```python
from build123d import *

# Parameters (mm, degrees)
F0_W     = 66.675
F0_H     = 125.4125
F0_W_2   = 63.5
F0_H_2   = 63.5
F1_DEPTH = 1.1811
F2_R     = 2.54
F2_R_2   = 6.35
F3_DEPTH = 1.1811
F4_R     = 5.08


with BuildPart() as f1:
    # F0 (on Top) → F1 (new body)
    with BuildSketch(Plane.XY):
        with Locations((0, 62.70625)):
            Rectangle(F0_W, F0_H)
        with Locations((-65.0875, 62.70625)):
            Rectangle(F0_W_2, F0_H)
        with Locations((65.0875, 62.70625)):
            Rectangle(F0_W_2, F0_H)
        with Locations((0, 157.1625)):
            Rectangle(F0_W, F0_H_2)
    extrude(amount=F1_DEPTH)

    # F2 (on face) → F3 (cut, through all)
    with BuildSketch(Plane.XY.offset(1.1811)):
        with BuildLine():
            ThreePointArc((-31.75, 109.5375), (-33.3375, 111.125), (-34.925, 109.5375))
            Line((-34.925, 109.5375), (-34.925, 90.4875))
            ThreePointArc((-34.925, 90.4875), (-33.3375, 88.9), (-31.75, 90.4875))
            Line((-31.75, 90.4875), (-31.75, 109.5375))
        make_face()
        with BuildLine():
            ThreePointArc((-31.75, 72.1995), (-33.3375, 73.787), (-34.925, 72.1995))
            Line((-34.925, 72.1995), (-34.925, 53.1495))
            ThreePointArc((-34.925, 53.1495), (-33.3375, 51.562), (-31.75, 53.1495))
            Line((-31.75, 53.1495), (-31.75, 72.1995))
        make_face()
        with BuildLine():
            ThreePointArc((-31.75, 34.8615), (-33.3375, 36.449), (-34.925, 34.8615))
            Line((-34.925, 34.8615), (-34.925, 15.8115))
            ThreePointArc((-34.925, 15.8115), (-33.3375, 14.224), (-31.75, 15.8115))
            Line((-31.75, 15.8115), (-31.75, 34.8615))
        make_face()
        with BuildLine():
            ThreePointArc((34.925, 34.8615), (33.3375, 36.449), (31.75, 34.8615))
            Line((31.75, 34.8615), (31.75, 15.8115))
            ThreePointArc((31.75, 15.8115), (33.3375, 14.224), (34.925, 15.8115))
            Line((34.925, 15.8115), (34.925, 34.8615))
        make_face()
        with BuildLine():
            ThreePointArc((34.925, 72.1995), (33.3375, 73.787), (31.75, 72.1995))
            Line((31.75, 72.1995), (31.75, 53.1495))
            ThreePointArc((31.75, 53.1495), (33.3375, 51.562), (34.925, 53.1495))
            Line((34.925, 53.1495), (34.925, 72.1995))
        make_face()
        with BuildLine():
            ThreePointArc((34.925, 109.5375), (33.3375, 111.125), (31.75, 109.5375))
            Line((31.75, 109.5375), (31.75, 90.4875))
            ThreePointArc((31.75, 90.4875), (33.3375, 88.9), (34.925, 90.4875))
            Line((34.925, 90.4875), (34.925, 109.5375))
        make_face()
        with BuildLine():
            ThreePointArc((-17.4625, 127), (-19.05, 125.4125), (-17.4625, 123.825))
            Line((-17.4625, 123.825), (-7.9375, 123.825))
            ThreePointArc((-7.9375, 123.825), (-6.35, 125.4125), (-7.9375, 127))
            Line((-7.9375, 127), (-17.4625, 127))
        make_face()
        with BuildLine():
            ThreePointArc((7.9375, 127), (6.35, 125.4125), (7.9375, 123.825))
            Line((7.9375, 123.825), (17.4625, 123.825))
            ThreePointArc((17.4625, 123.825), (19.05, 125.4125), (17.4625, 127))
            Line((17.4625, 127), (7.9375, 127))
        make_face()
        with Locations((-33.3375, 125.4125)):
            Circle(F2_R)
        with Locations((33.3375, 125.4125)):
            Circle(F2_R)
        with Locations((0, 74.6125)):
            Circle(F2_R_2)
    extrude(amount=-F3_DEPTH, mode=Mode.SUBTRACT)

    # F4
    f4_edges = [f1.edges().sort_by_distance(p)[0] for p in [
        (-96.8375, 0, 0.59055),
        (96.8375, 0, 0.59055),
    ]]
    fillet(f4_edges, radius=F4_R)


solid = f1.part
```
Read the model definition and answer for the solid it produces. Units are mm, in the model's axes. Coordinates: 2 decimals unless noted, no trailing zeros. Loops run counter-clockwise (first coordinate to the right, second up) from the corner with the lowest first, then second, coordinate; pieces in that order, holes last. Notation, with made-up numbers: (26.25, 81.5) -> (53.25, 81.5) arc R28 cw to (53.25, 109.5) -> close; hole circle Ø3 at (82.25, 40). An arc over 180 degrees is marked (long way). Return JSON: item names as keys, results as strings.
Item 1: Find section B-B (y = 77). Determine the outline of the cut face in (x, z).
Answers:
{"outline": "(-96.84, 0) -> (-5.88, 0) -> (-5.88, 1.18) -> (-96.84, 1.18) -> close; (5.88, 0) -> (96.84, 0) -> (96.84, 1.18) -> (5.88, 1.18) -> close"}
Item 2: Find section C-C (x = 78). Determine the outline of the cut face in (y, z), plus the area to 3 significant figures.
Answers:
{"outline": "(0, 0) -> (125.41, 0) -> (125.41, 1.18) -> (0, 1.18) -> close", "area": "148 mm2"}
Item 3: For a pull along X with two mould halves and no side action, classify faces 1 (the flat face through (-1, 96, 0)), 2 (the cylindrical face through (95.39, 1.53, 0.6)), 3 (the cylindrical face through (-95.39, 1.53, 0.6)), 4 (the cylindrical face through (3.41, 79.97, 0.6)) as +X half, -X half, draft (parallel to the pull), parting line (faces both ways), or undercut.
Answers:
{"face 1": "draft", "face 2": "+X half", "face 3": "-X half", "face 4": "undercut"}
Item 4: Flat-ended cylindrical pins translate along their axes: P1, Ø20.5, axis at x = 0, y = 74.61, coming from the -Z side; P2, Ø0.6, axis at x = -69, z = 0.5, coming from the +Y side. Find the tip coordinate at first contact, or state that the pin passes through.
Answers:
{"P1": "stops at z = 0", "P2": "stops at y = 125.41"}
Item 5: Find the intervals of material crossed by probe 1 along Y at (x, z) = (33.5, 1); probe 2 along Y at (x, z) = (0, 0.8); probe 3 along Y at (x, z) = (-85, 1.15), in increasing order.
Answers:
{"probe 1": "y = 0 to 14.23, 36.44 to 51.57, 73.78 to 88.91, 111.12 to 122.88", "probe 2": "y = 0 to 68.26, 80.96 to 188.91", "probe 3": "y = 0 to 125.41"}
Item 6: Find section D-D (z = 0.5). Count the separate pieces of the cut face and the enclosed holes in it, plus the area to 3 significant figures.
Answers:
{"separate pieces": "1", "enclosed holes": "9", "area": "27,900 mm2"}
Item 7: Find section A-A (x = 0). Determine the outline of the cut face in (y, z), plus the area to 3 significant figures.
Answers:
{"outline": "(0, 0) -> (68.26, 0) -> (68.26, 1.18) -> (0, 1.18) -> close; (80.96, 0) -> (188.91, 0) -> (188.91, 1.18) -> (80.96, 1.18) -> close", "area": "208 mm2"}
